Here's the drawing with two shaded views (mm, measured from the low corner). I have some questions. A direction names the side the tool comes from. Give positions to 0.01 mm unless a question says otherwise; leave off trailing zeros. Write each loop counter-clockwise with the first axis right and the second up, starting at its lowest first coordinate (ties: lowest second). Pieces come first, ordered by that corner, then holes. Notation, with made-up numbers: M 54.5,-25 L 78.5,-25 A6 cw 78.5,-21 Z; hole C -22.5,-26 d8. An arc over 180 degrees is marked long. Use one line per item in the form item = value.
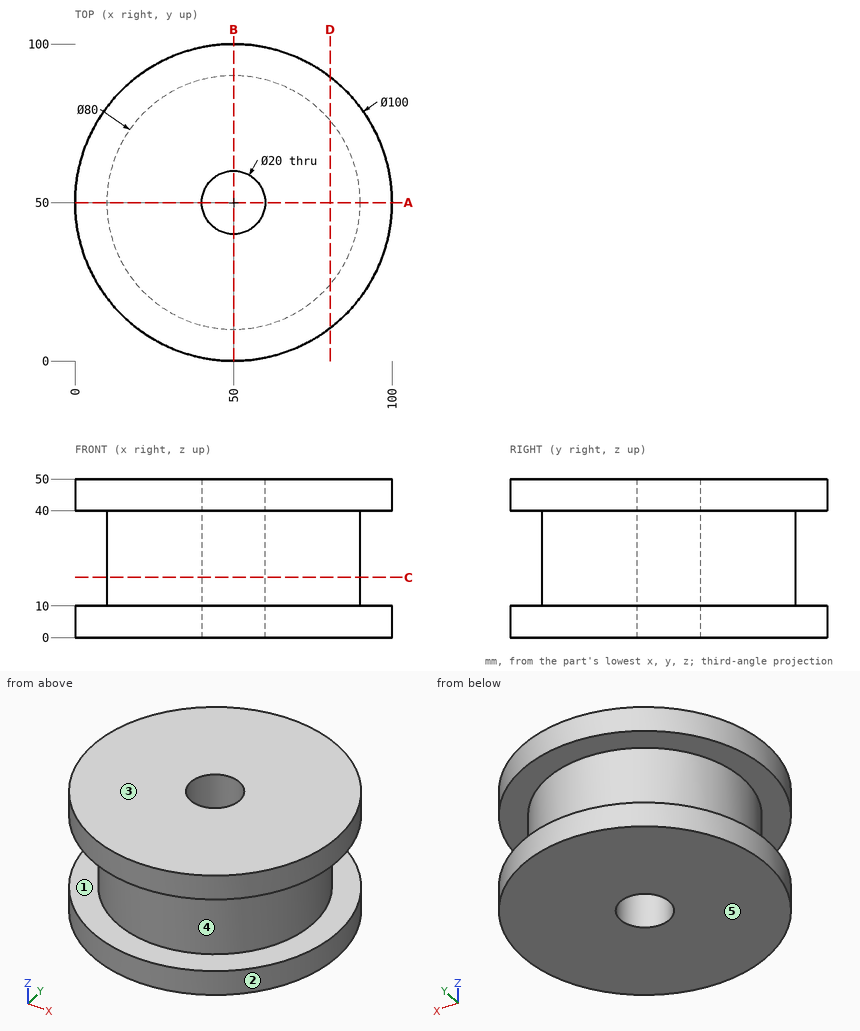
1) For the marked faces 4 and 5, which set-ups out of +Z, -Z, +X, -X, +Y, -Y let a thin tool reach every point of the face, with its end or its side?
Checked values:
face_4 = none
face_5 = -Z, +X, -X, +Y, -Y
2) I want a section at A-A, the plane y = 50. Please give me the cut outline in (x, z).
Checked values:
outline = M 0,0 L 40,0 L 40,50 L 0,50 L 0,40 L 10,40 L 10,10 L 0,10 Z; M 60,0 L 100,0 L 100,10 L 90,10 L 90,40 L 100,40 L 100,50 L 60,50 Z
3) I want a section at D-D, the plane x = 80.5. Please give me the cut outline in (y, z).
Checked values:
outline = M 10.38,0 L 89.62,0 L 89.62,10 L 75.88,10 L 75.88,40 L 89.62,40 L 89.62,50 L 10.38,50 L 10.38,40 L 24.12,40 L 24.12,10 L 10.38,10 Z
4) If I drill on L1, parallel to Z at x = 25, y = 85; L2, parallel to Y at x = 50, z = 12; L3, parallel to X at y = 41, z = 48, over which ranges is the centre line in solid material (lowest first)?
Checked values:
L1 = 0 to 10, 40 to 50
L2 = 10 to 40, 60 to 90
L3 = 0.82 to 45.64, 54.36 to 99.18
5) Thinking about a two-plate mould opening in Z: for the marked faces 1, 2 and 3, which applies, released by +Z, released by -Z, zero draft, split by the parting line, or undercut?
Checked values:
face_1 = undercut
face_2 = zero draft
face_3 = released by +Z
6) For pin 1 Ø1 at (y, z) = (62, 26.5) entering from +X; pin 2 Ø12 at (y, z) = (82.5, 6) entering from +X; pin 3 Ø4 at (y, z) = (89.5, 41) entering from -X, each with a flat end and sliding along its axis, tell me the tip position at first contact or that it passes through.
Checked values:
pin_1 = 88.31
pin_2 = 92.4
pin_3 = 16.93
7) I want a section at C-C, the plane z = 19. Please give me the cut outline in (x, y).
Checked values:
outline = C 50,50 d80; hole C 50,50 d20
